```python
from build123d import *

# Parameters (mm, degrees)
SKETCH1_R           = 0.5
SKETCH1_W           = 5
SKETCH1_H           = 5
SKETCH1_W_2         = 3.5
SKETCH1_H_2         = 3.5
BOSS_EXTRUDE3_DEPTH = 1
BOSS_EXTRUDE4_DEPTH = 0.4
CHAMFER1_SIZE       = 0.4
SKETCH5_R           = 1.5
BOSS_EXTRUDE5_DEPTH = 1
SKETCH6_R           = 1
CUT_EXTRUDE1_DEPTH  = 1


with BuildPart() as part:
    # Sketch1 → Boss-Extrude3 (new body)
    # profile 1 of 9: a face of its own
    with BuildSketch(Plane(origin=(0, 0, 0), x_dir=(1, 0, 0), z_dir=(0, 1, 0))):
        with Locations((-4.596194078, 4.596194078)):
            Circle(SKETCH1_R)
    # profile 2 of 9: a face of its own
    with BuildSketch(Plane(origin=(0, 0, 0), x_dir=(1, 0, 0), z_dir=(0, 1, 0))):
        with BuildLine():
            Line((-4.949747468, 4.242640687), (-2.5, 1.792893219))
            Line((-2.5, 1.792893219), (-2.5, 2.5))
            Line((-2.5, 2.5), (-1.792893219, 2.5))
            Line((-1.792893219, 2.5), (-4.242640687, 4.949747468))
            ThreePointArc((-4.242640687, 4.949747468), (-4.134254311, 4.787535794), (-4.096194078, 4.596194078))
            ThreePointArc((-4.096194078, 4.596194078), (-4.404852362, 4.134254311), (-4.949747468, 4.242640687))
        make_face()
    # profile 3 of 9: a face of its own
    with BuildSketch(Plane(origin=(0, 0, 0), x_dir=(1, 0, 0), z_dir=(0, 1, 0))):
        Rectangle(SKETCH1_W, SKETCH1_H)
        Rectangle(SKETCH1_W_2, SKETCH1_H_2, mode=Mode.SUBTRACT)
    # profile 4 of 9: a face of its own
    with BuildSketch(Plane(origin=(0, 0, 0), x_dir=(1, 0, 0), z_dir=(0, 1, 0))):
        with BuildLine():
            Line((2.5, 2.5), (2.5, 1.792893219))
            Line((2.5, 1.792893219), (4.949747468, 4.242640687))
            ThreePointArc((4.949747468, 4.242640687), (4.242640687, 4.242640687), (4.242640687, 4.949747468))
            Line((4.242640687, 4.949747468), (1.792893219, 2.5))
            Line((1.792893219, 2.5), (2.5, 2.5))
        make_face()
    # profile 5 of 9: a face of its own
    with BuildSketch(Plane(origin=(0, 0, 0), x_dir=(1, 0, 0), z_dir=(0, 1, 0))):
        with Locations((4.596194078, 4.596194078)):
            Circle(SKETCH1_R)
    # profile 6 of 9: a face of its own
    with BuildSketch(Plane(origin=(0, 0, 0), x_dir=(1, 0, 0), z_dir=(0, 1, 0))):
        with Locations((4.596194078, -4.596194078)):
            Circle(SKETCH1_R)
    # profile 7 of 9: a face of its own
    with BuildSketch(Plane(origin=(0, 0, 0), x_dir=(1, 0, 0), z_dir=(0, 1, 0))):
        with BuildLine():
            Line((2.5, -2.5), (1.792893219, -2.5))
            Line((1.792893219, -2.5), (4.242640687, -4.949747468))
            ThreePointArc((4.242640687, -4.949747468), (4.242640687, -4.242640687), (4.949747468, -4.242640687))
            Line((4.949747468, -4.242640687), (2.5, -1.792893219))
            Line((2.5, -1.792893219), (2.5, -2.5))
        make_face()
    # profile 8 of 9: a face of its own
    with BuildSketch(Plane(origin=(0, 0, 0), x_dir=(1, 0, 0), z_dir=(0, 1, 0))):
        with BuildLine():
            Line((-1.792893219, -2.5), (-2.5, -2.5))
            Line((-2.5, -2.5), (-2.5, -1.792893219))
            Line((-2.5, -1.792893219), (-4.949747468, -4.242640687))
            ThreePointArc((-4.949747468, -4.242640687), (-4.404852362, -4.134254311), (-4.096194078, -4.596194078))
            ThreePointArc((-4.096194078, -4.596194078), (-4.134254311, -4.787535794), (-4.242640687, -4.949747468))
            Line((-4.242640687, -4.949747468), (-1.792893219, -2.5))
        make_face()
    # profile 9 of 9: a face of its own
    with BuildSketch(Plane(origin=(0, 0, 0), x_dir=(1, 0, 0), z_dir=(0, 1, 0))):
        with Locations((-4.596194078, -4.596194078)):
            Circle(SKETCH1_R)
    extrude(amount=BOSS_EXTRUDE3_DEPTH)

    # Sketch4 → Boss-Extrude4 (add)
    with BuildSketch(Plane(origin=(0, 1, 0), x_dir=(1, 0, 0), z_dir=(0, 1, 0))):
        Polygon((-1.75, 0.875), (-0.875, 1.75), (-1.75, 1.75), align=None)
        Polygon((1.75, -0.875), (1.75, -1.75), (0.875, -1.75), align=None)
        Polygon((0.875, 1.75), (1.75, 0.875), (1.75, 1.75), align=None)
        Polygon((-0.875, -1.75), (-1.75, -1.75), (-1.75, -0.875), align=None)
    extrude(amount=-BOSS_EXTRUDE4_DEPTH)

    # Chamfer1
    chamfer1_edges = [part.edges().sort_by_distance(p)[0] for p in [
        (-1.75, 1, 0),
    ]]
    chamfer(chamfer1_edges, length=CHAMFER1_SIZE)

    # Sketch5 → Boss-Extrude5 (add)
    with BuildSketch(Plane(origin=(0, 1, 0), x_dir=(1, 0, 0), z_dir=(0, 1, 0))):
        with Locations((-3.889087297, 3.889087297)):
            Circle(SKETCH5_R)
        with Locations((3.889087297, -3.889087297)):
            Circle(SKETCH5_R)
        with Locations((3.889087297, 3.889087297)):
            Circle(SKETCH5_R)
        with Locations((-3.889087297, -3.889087297)):
            Circle(SKETCH5_R)
    extrude(amount=-BOSS_EXTRUDE5_DEPTH)

    # Sketch6 → Cut-Extrude1 (cut)
    with BuildSketch(Plane(origin=(0, 1, 0), x_dir=(1, 0, 0), z_dir=(0, 1, 0))):
        with Locations(Location((-3.889087297, 3.889087297, 0), (0, 0, 270))):
            Circle(SKETCH6_R)
        with Locations(Location((3.889087297, -3.889087297, 0), (0, 0, 90))):
            Circle(SKETCH6_R)
        with Locations(Location((3.889087297, 3.889087297, 0), (0, 0, 270))):
            Circle(SKETCH6_R)
        with Locations(Location((-3.889087297, -3.889087297, 0), (0, 0, 90))):
            Circle(SKETCH6_R)
    extrude(amount=-CUT_EXTRUDE1_DEPTH, mode=Mode.SUBTRACT)


solid = part.part
```
Build history of the part. All positions in model axes, mm. A direction names the side the tool comes from. Round coordinates to 2 decimals unless told otherwise and drop trailing zeros. Loops run counter-clockwise (first coordinate to the right, second up) from the corner with the lowest first, then second, coordinate; pieces in that order, holes last. Notation, with made-up numbers: M 52.25,36 L 76.25,36 A16 cw 76.25,51 Z; hole C 76.5,-15 d7. An arc over 180 degrees is marked long. Answer as CSV lines item,"result".
1. Flat gauge pins, fed straight in: P1, Ø1.8, axis at x = -3.89, z = -3.89, coming from the +Y side; P2, Ø0.5, axis at x = -0.5, y = 0.5, coming from the -Z side. Where does each tip first touch, or does it go through?
Resolved:
P1,"passes through"
P2,"stops at z = -2.5"
2. Cut at A-A on z = 0. Write the cut outline in (x, y).
Resolved:
outline,"M -2.5,0 L -1.75,0 L -1.75,0.6 L -2.15,1 L -2.5,1 Z; M 1.75,0 L 2.5,0 L 2.5,1 L 1.75,1 Z"
3. Cut at C-C on z = 4.5. Write the cut outline in (x, y), then the cut area to 3 significant figures.
Resolved:
outline,"M -5.26,0 L -4.68,0 L -4.68,1 L -5.26,1 Z; M -3.1,0 L -2.52,0 L -2.52,1 L -3.1,1 Z; M 2.52,0 L 3.1,0 L 3.1,1 L 2.52,1 Z; M 4.68,0 L 5.26,0 L 5.26,1 L 4.68,1 Z"
area,"2.31 mm²"
4. Cut at B-B on x = 1. Write the cut outline in (y, z) (3 decimals), then the cut area to 3 significant figures.
Resolved:
outline,"M 0,-2.5 L 1,-2.5 L 1,-1.625 L 0.6,-1.625 L 0.6,-1.75 L 0,-1.75 Z; M 0,1.75 L 0.6,1.75 L 0.6,1.625 L 1,1.625 L 1,2.5 L 0,2.5 Z"
area,"1.60 mm²"
5. Cut at D-D on y = 0.2. Write the cut outline in (x, z), then the cut area to 3 significant figures.
Resolved:
outline,"M -3.24,-2.54 A1.5 ccw long -2.54,-3.24 L -1.79,-2.5 L 1.79,-2.5 L 2.54,-3.24 A1.5 ccw long 3.24,-2.54 L 2.5,-1.79 L 2.5,1.79 L 3.24,2.54 A1.5 ccw long 2.54,3.24 L 1.79,2.5 L -1.79,2.5 L -2.54,3.24 A1.5 ccw long -3.24,2.54 L -2.5,1.79 L -2.5,-1.79 Z; hole C -3.89,-3.89 d2; hole C -3.89,3.89 d2; hole M -1.75,-1.75 L 1.75,-1.75 L 1.75,1.75 L -1.75,1.75 Z; hole C 3.89,-3.89 d2; hole C 3.89,3.89 d2"
area,"31.4 mm²"
6. Wall check: probe 1 along X at (y, z) = (0.6, 3); probe 2 along X at (y, z) = (0.2, -0.5); probe 3 along Z at (x, y) = (-3.75, 0.1). Give the ranges that are in metal, low to high. Write a range as [from, to].
Resolved:
probe 1,"x = [-5.1, -4.35], [-3.43, -2.29], [2.29, 3.43], [4.35, 5.1]"
probe 2,"x = [-2.5, -1.75], [1.75, 2.5]"
probe 3,"z = [-5.38, -4.88], [-2.9, -2.4], [2.4, 2.9], [4.88, 5.38]"
7. 3-axis set-ups, long thin cutter, end or side, ignore diameter. For faces 1 (the flat face through (1.5, 0.6, 1.5)), 2 (the flat face through (0, 0, 2)), 3 (the flat face through (1.306, 0.803, 1.319)), 4 (the flat face through (-1.38, 0.803, 1.245)): which of +Z, -Z, +X, -X, +Y, -Y reach the whole face in a straight line?
Resolved:
face 1,"-Y"
face 2,"+Z, -Z, +X, -X, -Y"
face 3,"+Y, -Y"
face 4,"+Y"
8. Two-plate mould, pull along Z, no slides. Class faces 5 (the flat face through (0, 0.5, -2.5)), 6 (the flat face through (-1.38, 0.803, -1.245)), 7 (the cylindrical face through (4.189, 0.507, -2.935)), 8 (the flat face through (0, 1, -2)): released by +Z, released by -Z, zero draft, split by the parting line, or undercut.
Resolved:
face 5,"released by -Z"
face 6,"undercut"
face 7,"undercut"
face 8,"zero draft"
